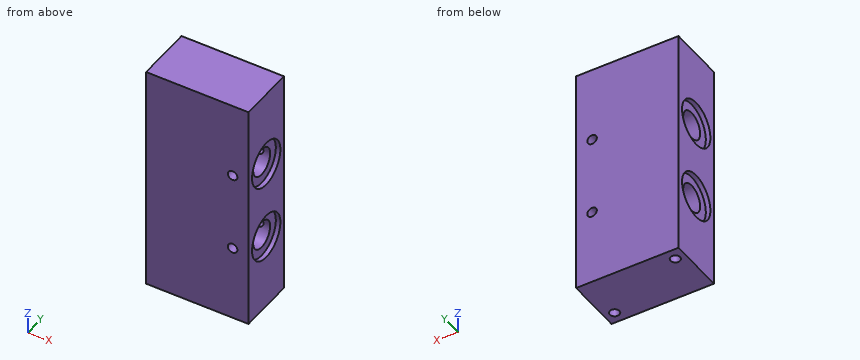
from build123d import *

# Parameters (mm, degrees)
SKETCH1_W             = 45
SKETCH1_H             = 102
BOSS_EXTRUDE1_DEPTH   = 25
M5_TAPPED_HOLE3_D     = 4.2
SKETCH27_R            = 6
CUT_EXTRUDE1_DEPTH    = 74
SKETCH28_R            = 10
CUT_EXTRUDE3_DEPTH    = 2
SKETCH30_R            = 10
CUT_EXTRUDE4_DEPTH    = 2
M5_TAPPED_HOLE4_D     = 4.2
M5_TAPPED_HOLE4_DEPTH = 14
M5_TAPPED_HOLE4_TIP   = 1.2618073


with BuildPart() as part:
    # Sketch1 → Boss-Extrude1 (new body)
    with BuildSketch(Plane(origin=(0, 0, 0), x_dir=(1, 0, 0), z_dir=(0, 1, 0))):
        Rectangle(SKETCH1_W, SKETCH1_H)
    extrude(amount=BOSS_EXTRUDE1_DEPTH)

    # M5 Tapped Hole3 (through all)
    with Locations(Plane(origin=(0, 25, 0), x_dir=(1, 0, 0), z_dir=(0, 1, 0))):
        with Locations((15.5, 17.5), (15.5, -17.5)):
            Hole(M5_TAPPED_HOLE3_D / 2)

    # Sketch27 → Cut-Extrude1 (cut)
    with BuildSketch(Plane.ZY.offset(22.5)):
        with Locations((-17.5, 12.5)):
            Circle(SKETCH27_R)
        with Locations((17.5, 12.5)):
            Circle(SKETCH27_R)
    extrude(amount=-CUT_EXTRUDE1_DEPTH, mode=Mode.SUBTRACT)

    # Sketch28 → Cut-Extrude3 (cut)
    with BuildSketch(Plane.ZY.offset(22.5)):
        with Locations((-17.5, 12.5)):
            Circle(SKETCH28_R)
        with Locations((17.5, 12.5)):
            Circle(SKETCH28_R)
    extrude(amount=-CUT_EXTRUDE3_DEPTH, mode=Mode.SUBTRACT)

    # Sketch30 → Cut-Extrude4 (cut)
    with BuildSketch(Plane(origin=(22.5, 0, 0), x_dir=(0, 0, -1), z_dir=(1, 0, 0))):
        with Locations((-17.5, 12.5)):
            Circle(SKETCH30_R)
        with Locations((17.5, 12.5)):
            Circle(SKETCH30_R)
    extrude(amount=-CUT_EXTRUDE4_DEPTH, mode=Mode.SUBTRACT)

    # M5 Tapped Hole4
    with Locations(Plane(origin=(0, 0, -51), x_dir=(-1, 0, 0), z_dir=(0, 0, -1))):
        with Locations((-18, 5), (18, 20)):
            Hole(M5_TAPPED_HOLE4_D / 2, depth=M5_TAPPED_HOLE4_DEPTH)
            with Locations((0, 0, -(M5_TAPPED_HOLE4_DEPTH + M5_TAPPED_HOLE4_TIP / 2))):  # 118° drill point
                Cone(0, M5_TAPPED_HOLE4_D / 2, M5_TAPPED_HOLE4_TIP, mode=Mode.SUBTRACT)


solid = part.part
CAD build for the part. Positions are in the model's coordinates, mm. Give positions to 0.01 mm unless a question says otherwise; leave off trailing zeros. Loops run counter-clockwise (first coordinate to the right, second up) from the corner with the lowest first, then second, coordinate; pieces in that order, holes last. Notation, with made-up numbers: M 67.25,-25 L 77.25,-25 A23 cw 77.25,-8 Z; hole C 0.5,2 d10. An arc over 180 degrees is marked long. One line per question, with ' | ' between items. Start each with the question number.
1. Flat gauge pin, fed straight in: pin 1 (2.5 mm diameter, centred on x = 18, y = 5, fed in from -Z). Where does the tip first touch, or does it go through?
2. Probe L1, parallel to Z at x = 15.5, y = 21; L2, parallel to Y at x = 18, z = -42.25; L3, parallel to X at y = 5, z = -45.5. List the from-to ranges inside material, lowest first. Write a range as from..to.
3. Saw through at B-B on z = -17.5. Give the cut face in (x, y), plus the area to 3 significant figures.
4. Saw through at A-A on y = 12.5. Give the cut face in (x, z), plus the area to 3 significant figures.
5. Saw through at C-C on x = -8.5. Give the cut face in (y, z), plus the area to 3 significant figures.
6. Saw through at D-D on y = 16.5. Give the cut face in (x, z).
Result sheet:
1) pin 1: stops at z = -36.49
2) L1: z = -51..-19.6, -15.4..15.4, 19.6..51 | L2: y = 0..2.9, 7.1..25 | L3: x = -22.5..15.9, 20.1..22.5
3) outline: M -22.5,0 L 13.4,0 L 13.4,6.5 L -20.5,6.5 L -20.5,2.5 L -22.5,2.5 Z; M -22.5,22.5 L -20.5,22.5 L -20.5,18.5 L 13.4,18.5 L 13.4,25 L -22.5,25 Z; M 17.6,0 L 22.5,0 L 22.5,2.5 L 20.5,2.5 L 20.5,6.5 L 17.6,6.5 Z; M 17.6,18.5 L 20.5,18.5 L 20.5,22.5 L 22.5,22.5 L 22.5,25 L 17.6,25 Z | area: 498 mm^2
4) outline: M -22.5,-51 L 22.5,-51 L 22.5,-27.5 L 20.5,-27.5 L 20.5,-23.5 L -20.5,-23.5 L -20.5,-27.5 L -22.5,-27.5 Z; M -22.5,-7.5 L -20.5,-7.5 L -20.5,-11.5 L 20.5,-11.5 L 20.5,-7.5 L 22.5,-7.5 L 22.5,7.5 L 20.5,7.5 L 20.5,11.5 L -20.5,11.5 L -20.5,7.5 L -22.5,7.5 Z; M -22.5,27.5 L -20.5,27.5 L -20.5,23.5 L 20.5,23.5 L 20.5,27.5 L 22.5,27.5 L 22.5,51 L -22.5,51 Z | area: 3,450 mm^2
5) outline: M 0,-51 L 25,-51 L 25,51 L 0,51 Z; hole C 12.5,-17.5 d12; hole C 12.5,17.5 d12 | area: 2,320 mm^2
6) outline: M -22.5,-51 L 22.5,-51 L 22.5,-26.67 L 20.5,-26.67 L 20.5,-21.97 L -20.5,-21.97 L -20.5,-26.67 L -22.5,-26.67 Z; M -22.5,-8.33 L -20.5,-8.33 L -20.5,-13.03 L 20.5,-13.03 L 20.5,-8.33 L 22.5,-8.33 L 22.5,8.33 L 20.5,8.33 L 20.5,13.03 L -20.5,13.03 L -20.5,8.33 L -22.5,8.33 Z; M -22.5,26.67 L -20.5,26.67 L -20.5,21.97 L 20.5,21.97 L 20.5,26.67 L 22.5,26.67 L 22.5,51 L -22.5,51 Z
